Geometry check sheet. Reference: drawing and pictorial views, mm from the part's lowest x, y, z. A direction names the side the tool comes from. Give positions to 0.01 mm unless a question says otherwise; leave off trailing zeros. Write each loop counter-clockwise with the first axis right and the second up, starting at its lowest first coordinate (ties: lowest second). Pieces come first, ordered by that corner, then holes. Notation, with made-up numbers: (46, 20.5) -> (50, 20.5) arc R18 ccw to (50, 41.5) -> close; hole circle Ø11 at (-21.5, 37.5). An arc over 180 degrees is marked (long way). Write each question's results on one line, items separated by ' | '. Start each with the question number.
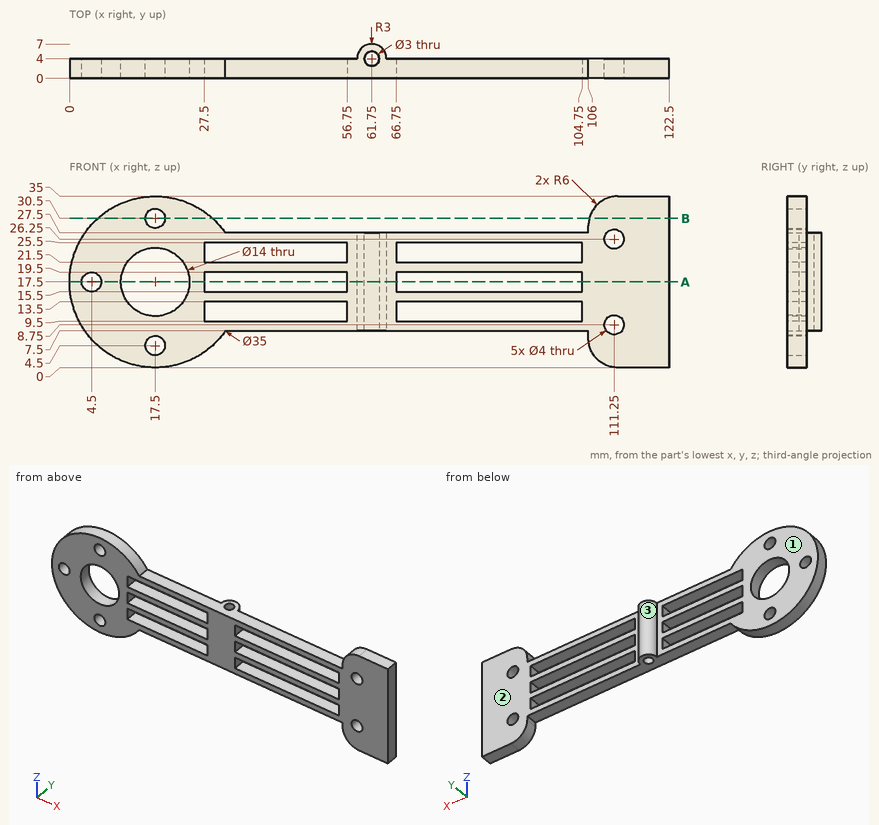
Item 1: Section check A-A on z = 17.5. Record the boundary of the cut face in (x, y).
Item 2: Thickness scan on probe 1 along Z at (x, y) = (89.5, 1.5); probe 2 along X at (y, z) = (4.25, 21); probe 3 along X at (y, z) = (2, 25). Record the ranges inside material, lowest first. Write a range as from..to.
Item 3: Depth check by flat-ended pin: pin 1 Ø3 at (x, y) = (35, 2.5) entering from +Z; pin 2 Ø3 at (x, y) = (37, 1.5) entering from -Z; pin 3 Ø1.5 at (y, z) = (5, 15) entering from -X; pin 4 Ø3 at (x, z) = (111.25, 26.25) entering from -Y. Enter the tip coordinate at first touch or a pass-through.
Item 4: Section check B-B on z = 30.5. Record the boundary of the cut face in (x, y).
Item 5: Set-up check for the marked faces 1, 2 and 3: record each of +Z, -Z, +X, -X, +Y, -Y from which the full face is reachable in a straight line by a thin tool's end or side.
Check sheet entries:
1) outline: (0, 0) -> (2.5, 0) -> (2.5, 4) -> (0, 4) -> close; (6.5, 0) -> (10.5, 0) -> (10.5, 4) -> (6.5, 4) -> close; (24.5, 0) -> (27.5, 0) -> (27.5, 4) -> (24.5, 4) -> close; (56.75, 0) -> (66.75, 0) -> (66.75, 4) -> (64.75, 4) arc R3 ccw to (58.75, 4) -> (56.75, 4) -> close; (104.75, 0) -> (122.5, 0) -> (122.5, 4) -> (104.75, 4) -> close; hole circle Ø3 at (61.75, 4)
2) probe 1: z = 7.5..9.5, 13.5..15.5, 19.5..21.5, 25.5..27.5 | probe 2: x = 58.76..60.27, 63.23..64.74 | probe 3: x = 1.69..27.5, 56.75..66.75, 104.75..109.69, 112.81..122.5
3) pin 1: stops at z = 27.5 | pin 2: stops at z = 7.5 | pin 3: stops at x = 58.76 | pin 4: passes through
4) outline: (5.78, 0) -> (15.5, 0) -> (15.5, 4) -> (5.78, 4) -> close; (19.5, 0) -> (29.22, 0) -> (29.22, 4) -> (19.5, 4) -> close; (106.19, 0) -> (122.5, 0) -> (122.5, 4) -> (106.19, 4) -> close
5) face 1: +Z, -Z, -X, +Y | face 2: +Z, -Z, +X, +Y | face 3: +Z, -Z, +Y
